from build123d import *

# Parameters (mm, degrees)
SKETCH_2_R          = 3
CUT_EXTRUDE_1_DEPTH = 15


with BuildPart() as part:
    # 草图1 → 旋转1 (revolve)
    with BuildSketch(Plane.XY):
        with BuildLine():
            Line((41, 16), (77, 16))
            ThreePointArc((77, 16), (78.414213562, 16.585786438), (79, 18))
            Line((79, 18), (79, 58))
            Line((79, 58), (87, 58))
            Line((87, 58), (88, 50))
            Line((88, 50), (116, 50))
            Line((116, 50), (117, 58))
            Line((117, 58), (125, 58))
            Line((125, 58), (125, 18))
            ThreePointArc((125, 18), (125.585786438, 16.585786438), (127, 16))
            Line((127, 16), (163, 16))
            Line((163, 16), (164, 15))
            Line((164, 15), (164, 12.5))
            Line((164, 12.5), (259, 12.5))
            Line((259, 12.5), (260, 11.5))
            Line((260, 11.5), (260, 0))
            Line((260, 0), (0, 0))
            Line((0, 0), (0, 11.5))
            Line((0, 11.5), (1, 12.5))
            Line((1, 12.5), (40, 12.5))
            Line((40, 12.5), (40, 15))
            Line((40, 15), (41, 16))
        make_face()
    revolve(axis=Axis((0, 0, 0), (1, 0, 0)))

    # 草图2 → 切除-拉伸1 (cut, symmetric)
    with BuildSketch(Plane.XY):
        with Locations((230, 0)):
            Circle(SKETCH_2_R)
    extrude(amount=CUT_EXTRUDE_1_DEPTH, both=True, mode=Mode.SUBTRACT)


solid = part.part
The listing builds one solid part. Answer for the finished solid, in the listing's coordinates (mm). A direction names the side the tool comes from. Give positions to 0.01 mm unless a question says otherwise; leave off trailing zeros. Write each loop counter-clockwise with the first axis right and the second up, starting at its lowest first coordinate (ties: lowest second). Pieces come first, ordered by that corner, then holes.
Item 1: Determine the mould class of faces 1 (the cylindrical face through (20.773, 11.923, 3.755)), 2 (the conical face through (116.063, -10.948, -49.3)), 3 (the flat face through (260, 0, 0)) for opening direction X: released by +X, released by -X, zero draft, split by the parting line, or undercut.
Item 2: Which of the six approach directions +Z, -Z, +X, -X, +Y, -Y give full straight-line access (tool end or side, diameter ignored) to faces 4 (the cylindrical face through (212.165, 11.923, 3.755)), 5 (the cylindrical face through (59.25, -3.47, -15.62)), 6 (the conical face through (87.95, -39.99, -30.66))?
Item 3: Flat-ended cylindrical pins translate along their axes: P1, Ø8, axis at y = 31, z = -44.5, coming from the -X side; P2, Ø5, axis at y = -43.5, z = 15.5, coming from the +X side; P3, Ø6, axis at x = 149, y = -0.5, coming from the -Z side. Find the tip coordinate at first contact, or state that the pin passes through.
Item 4: Section B-B, the plane x = 44 is taken. Write down the section's boundary in (y, z), plus the area to 3 significant figures.
Item 5: Find the intervals of material crossed by line 1 along X through (y, z) = (0, 0); line 2 along Y through (x, z) = (230, -0.75); line 3 along Y through (x, z) = (230, 5), in increasing order.
Item 6: Section A-A, the plane x = 208.5 is taken. Write down the section's boundary in (y, z).
Completed:
1. face 1: zero draft
1. face 2: undercut
1. face 3: released by +X
2. face 4: +X
2. face 5: -X
2. face 6: none
3. P1: stops at x = 79
3. P2: stops at x = 125
3. P3: stops at z = -16
4. outline: circle Ø32 at (0, 0)
4. area: 804 mm2
5. line 1: x = 0 to 227, 233 to 260
5. line 2: y = -12.48 to -3, 3 to 12.48
5. line 3: y = -11.46 to -3, 3 to 11.46
6. outline: circle Ø25 at (0, 0)
